Job drawing, mm, ordinate dimensions from the low corner. One solid piece. A direction names the side the tool comes from. Give positions to 0.01 mm unless a question says otherwise; leave off trailing zeros. Loops run counter-clockwise (first coordinate to the right, second up) from the corner with the lowest first, then second, coordinate; pieces in that order, holes last. Notation, with made-up numbers: (58.5, 69.5) -> (64.5, 69.5) arc R34 ccw to (64.5, 107.5) -> close; hole circle Ø5 at (19, -12.5). An arc over 180 degrees is marked (long way). Answer as a JSON object with one key per item and string values. Group by question number.
Q1. Wall check: probe 1 along Z at (x, y) = (14.75, 10.5); probe 2 along Z at (x, y) = (12, 10.25); probe 3 along Y at (x, z) = (11.75, 18.25). Give the ranges that are in metal, low to high. Write a range as from..to.
Q2. Drop flat-ended pins along their axis: pin 1 (4 mm diameter, centred on y = 12.5, z = 4, fed in from +X); pin 2 (3 mm diameter, centred on y = 8.5, z = 12.5, fed in from +X); pin 3 (6.5 mm diameter, centred on x = 17, y = 9.5, fed in from +Z); pin 4 (1.5 mm diameter, centred on y = 10.5, z = 12.5, fed in from -X). Give the stop position or say it passes through.
Q3. Tool access for the marked faces 1 and 2: list every direction of +Z, -Z, +X, -X, +Y, -Y with a clear straight run to the whole face (end or side of a thin tool).
Q4. Band-saw the part on C-C, the plane z = 6.25. Write the cut outline in (x, y).
Q5. Band-saw the part on A-A, the plane y = 12. Write the cut outline in (x, z).
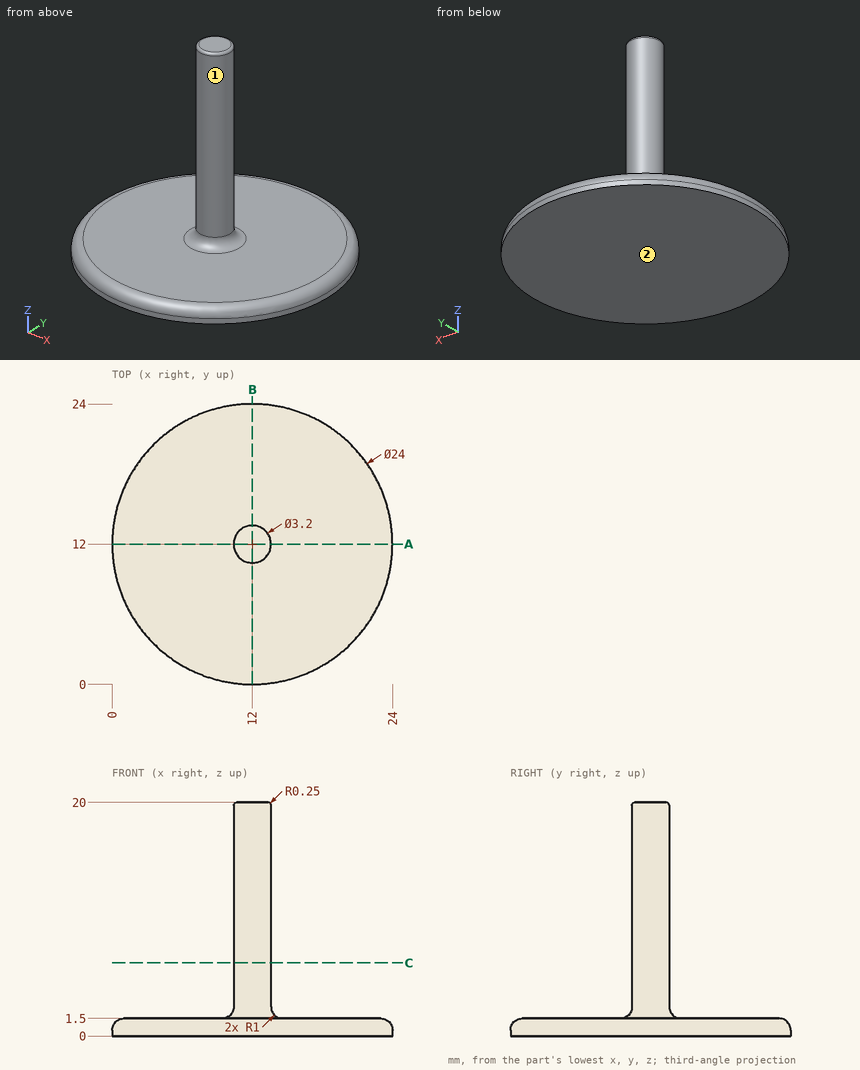
Worked answers:
{
 "1": {"probe 1": "0..1.5", "probe 2": "0..1.97", "probe 3": "10.42..13.58"},
 "2": {"pin 1": "x = 13.71", "pin 2": "through", "pin 3": "z = 1.53", "pin 4": "x = 10.59"},
 "3": {"face 1": "+Z", "face 2": "-Z, +X, -X, +Y, -Y"},
 "4": {"outline": "circle Ø3.2 at (12, 12)"},
 "5": {"outline": "(0, 0) -> (24, 0) -> (24, 0.5) arc R1 ccw to (23, 1.5) -> (14.6, 1.5) arc R1 cw to (13.6, 2.5) -> (13.6, 19.75) arc R0.25 ccw to (13.35, 20) -> (10.65, 20) arc R0.25 ccw to (10.4, 19.75) -> (10.4, 2.5) arc R1 cw to (9.4, 1.5) -> (1, 1.5) arc R1 ccw to (0, 0.5) -> close"}
}
